Input: part model. Units: mm. Frame: model coordinates. A direction names the side the tool comes from. Coordinates: 2 decimals unless noted, no trailing zeros. Loops run counter-clockwise (first coordinate to the right, second up) from the corner with the lowest first, then second, coordinate; pieces in that order, holes last. Notation, with made-up numbers: (17.25, -34) -> (71.25, -34) arc R16 cw to (71.25, -8) -> close; hole circle Ø1 at (61.5, -10). An arc over 180 degrees is marked (long way). Answer as a JSON object with one key per item and string values.
from build123d import *

# Parameters (mm, degrees)
BOSS_EXTRUDE1_DEPTH  = 13
CUT_EXTRUDE1_DEPTH   = 66.5
BOSS_EXTRUDE4_DEPTH  = 6.1
CUT_EXTRUDE2_DEPTH   = 6.1
BOSS_EXTRUDE6_DEPTH  = 2.5
BOSS_EXTRUDE7_DEPTH  = 2.5
BOSS_EXTRUDE8_DEPTH  = 19.1
BOSS_EXTRUDE12_DEPTH = 9.5
BOSS_EXTRUDE13_DEPTH = 2.5
CUT_EXTRUDE4_DEPTH   = 5
CUT_EXTRUDE5_DEPTH   = 6.5
BOSS_EXTRUDE14_DEPTH = 10
CUT_EXTRUDE7_DEPTH   = 13
CUT_EXTRUDE8_DEPTH   = 5
CUT_EXTRUDE9_DEPTH   = 5
BOSS_EXTRUDE15_DEPTH = 2


with BuildPart() as part:
    # 3DSketch1 → Boss-Extrude1 (new body)
    with BuildSketch(Plane(origin=(0, 0, 0), x_dir=(0.970570246541768, 0, 0.2408181814727695), z_dir=(0, 1, 0))):
        Polygon((0, 0), (64.542921395, 16.014409068), (68.516421389, 0), (3.973499994, -16.014409068), align=None)
    extrude(amount=BOSS_EXTRUDE1_DEPTH)

    # 3DSketch2 → Cut-Extrude1 (cut)
    with BuildSketch(Plane(origin=(0, 13, 3.5), x_dir=(0, -0.8073911222578979, 0.59001658934231), z_dir=(1, 0, 0))):
        Polygon((0, 0), (10.496084589, 7.670215661), (11.971126063, 5.651737856), (1.475041473, -2.018477806), align=None)
        Polygon((14.626200715, 2.018477806), (4.130116125, -5.651737856), (5.605157599, -7.670215661), (16.101242188, 0), align=None)
    extrude(amount=CUT_EXTRUDE1_DEPTH, mode=Mode.SUBTRACT)


with BuildPart() as cut_extrude1_piece_1:
    # of the separate pieces the step leaves, piece 1, a body of its own (cut_extrude1_pieces)
    add(part.part.solids().sort_by_distance((0, 0, 10.5))[0])



with BuildPart() as cut_extrude1_piece_2:
    # of the separate pieces the step leaves, piece 2, a body of its own (cut_extrude1_pieces)
    add(part.part.solids().sort_by_distance((0, 0, 16.5))[0])


with BuildPart() as cut_extrude1_piece_3:
    # of the separate pieces the step leaves, piece 3, a body of its own (cut_extrude1_pieces)
    add(part.part.solids().sort_by_distance((0, 0, 0))[0])


with BuildPart() as cut_extrude1_piece_1_1:
    add(cut_extrude1_piece_1.part)

    add(cut_extrude1_piece_2.part)  # Boss-Extrude4 merges Cut-Extrude1 piece 2

    add(cut_extrude1_piece_3.part)  # Boss-Extrude4 merges Cut-Extrude1 piece 3
    # 3DSketch3 → Boss-Extrude4 (add)
    with BuildSketch(Plane(origin=(0, 13, 0), x_dir=(0.970570246541768, 0, 0.2408181814727695), z_dir=(0, 1, 0))):
        Polygon((0, 0), (64.542921395, 16.014409068), (68.516421389, 0), (3.973499994, -16.014409068), align=None)
    extrude(amount=BOSS_EXTRUDE4_DEPTH)

    # 3DSketch4 → Cut-Extrude2 (cut)
    with BuildSketch(Plane(origin=(2.463625992, 19.1, 3.5), x_dir=(0.9882657761690827, 0, 0.15274408549243565), z_dir=(0, 1, 0))):
        Polygon((0, 0), (60.744465433, 9.388524874), (62.195534245, 0), (1.451068812, -9.388524874), align=None)
    extrude(amount=-CUT_EXTRUDE2_DEPTH, mode=Mode.SUBTRACT)

    # 3DSketch5 → Boss-Extrude6 (add)
    with BuildSketch(Plane(origin=(0, 13, 3.5), x_dir=(0, -0.38512437764181645, 0.9228646779165425), z_dir=(-1, 0, 0))):
        Polygon((0, 0), (0.564008213, -1.351519893), (1.526819157, -3.658681588), (3.833980852, -2.695870643), (2.871169908, -0.388708949), (2.307161695, 0.962810944), align=None)
        Polygon((6.460052745, 2.695870643), (7.024060958, 1.344350751), (7.986871902, -0.962810944), (10.294033597, 0), (9.331222653, 2.307161695), (8.76721444, 3.658681588), align=None)
    extrude(amount=-BOSS_EXTRUDE6_DEPTH)

    # 3DSketch6 → Boss-Extrude7 (add)
    with BuildSketch(Plane(origin=(66.5, 0, 13), x_dir=(0, 0.8073911222578979, -0.5900165893423102), z_dir=(-1, 0, 0))):
        Polygon((0, 0), (1.475041473, 2.018477806), (11.971126063, -5.651737856), (10.496084589, -7.670215661), align=None)
        Polygon((14.626200715, -2.018477806), (4.130116125, 5.651737856), (5.605157599, 7.670215661), (16.101242188, 0), align=None)
    extrude(amount=BOSS_EXTRUDE7_DEPTH)

    # 3DSketch7 → Boss-Extrude8 (add)
    with BuildSketch(Plane(origin=(66.5, 0, 0), x_dir=(0.7713732785400773, 0, 0.6363829547955637), z_dir=(0, 1, 0))):
        Polygon((0, 0), (15.427465571, 12.727659096), (25.927784325, 0), (10.500318754, -12.727659096), align=None)
    extrude(amount=BOSS_EXTRUDE8_DEPTH)

    # 3DSketch8 → Boss-Extrude12 (add)
    with BuildSketch(Plane(origin=(76.128891267, 13, 6), x_dir=(-0.9382075830120803, 0, 0.3460730142305674), z_dir=(0, 1, 0))):
        Polygon((0, 0), (1.557328564, 4.221934124), (-1.734607538, 5.436217903), (-3.291936102, 1.214283779), align=None)
    extrude(amount=BOSS_EXTRUDE12_DEPTH)

    # 3DSketch9 → Boss-Extrude13 (add)
    with BuildSketch(Plane(origin=(75.345809824, 22.5, 11.764688466), x_dir=(0.5846855732237681, 0, -0.8112599956018993), z_dir=(0, 1, 0))):
        Polygon((0, 0), (5.702652298, 4.10997528), (8.664764649, 0), (2.962112351, -4.10997528), align=None)
    extrude(amount=BOSS_EXTRUDE13_DEPTH)

    # 3DSketch11 → Cut-Extrude4 (cut)
    with BuildSketch(Plane(origin=(0, 0, 0), x_dir=(0.9822888340033693, 0, 0.18737301457867736), z_dir=(0, -1, 0))):
        Polygon((0, 0), (3.091654741, 16.207765761), (88.059638882, 0), (84.967984141, -16.207765761), align=None)
    extrude(amount=-CUT_EXTRUDE4_DEPTH, mode=Mode.SUBTRACT)

    # 3DSketch12 → Cut-Extrude5 (cut)
    with BuildSketch(Plane(origin=(86.5, 5, 0), x_dir=(0, 0.6496523275821462, 0.7602314471705968), z_dir=(1, 0, 0))):
        Polygon((0, 0), (12.543818878, 10.719263405), (21.703916697, 0), (9.160097819, -10.719263405), align=None)
    extrude(amount=-CUT_EXTRUDE5_DEPTH, mode=Mode.SUBTRACT)

    # 3DSketch13 → Boss-Extrude14 (add)
    with BuildSketch(Plane(origin=(79.637641528, 22.5, 10.5), x_dir=(0, -0.6028330891856902, -0.7978673239222407), z_dir=(-1, 0, 0))):
        Polygon((0, 0), (2.049632503, 2.712748901), (5.640035461, 0), (3.590402958, -2.712748901), align=None)
    extrude(amount=BOSS_EXTRUDE14_DEPTH)

    # 3DSketch14 → Cut-Extrude7 (cut)
    with BuildSketch(Plane(origin=(80.41197271, 22.5, 4.735311534), x_dir=(0, 0.3350889131315588, 0.9421865103557314), z_dir=(-1, 0, 0))):
        Polygon((0, 0), (0.837722283, 2.355466276), (7.460706404, 0), (6.622984121, -2.355466276), align=None)
    extrude(amount=CUT_EXTRUDE7_DEPTH, mode=Mode.SUBTRACT)

    # 3DSketch15 → Cut-Extrude8 (cut)
    with BuildSketch(Plane(origin=(79.637641528, 22.5, 10.5), x_dir=(0, -0.6028330891856902, -0.7978673239222407), z_dir=(-1, 0, 0))):
        Polygon((0, 0), (2.049632503, 2.712748901), (5.640035461, 0), (3.590402958, -2.712748901), align=None)
    extrude(amount=CUT_EXTRUDE8_DEPTH, mode=Mode.SUBTRACT)

    # 3DSketch16 → Cut-Extrude9 (cut)
    with BuildSketch(Plane(origin=(80, 19.1, 0), x_dir=(0, -0.6496523275821462, 0.7602314471705968), z_dir=(-1, 0, 0))):
        Polygon((0, 0), (12.543818878, 10.719263405), (21.703916697, 0), (9.160097819, -10.719263405), align=None)
    extrude(amount=CUT_EXTRUDE9_DEPTH, mode=Mode.SUBTRACT)

    # 3DSketch17 → Boss-Extrude15 (add)
    with BuildSketch(Plane(origin=(68.168662732, 22.5, 12.3202178), x_dir=(0.6981467055639471, 0, -0.7159547314671559), z_dir=(0, -1, 0))):
        Polygon((0, 0), (5.828183385, -5.683218296), (11.370042327, 0), (5.541858942, 5.683218296), align=None)
    extrude(amount=-BOSS_EXTRUDE15_DEPTH)


solid = cut_extrude1_piece_1_1.part
1. Section query A-A (x = 31). Return loops of the section in (y, z), plus the area to 3 significant figures.
Reply:
{"outline": "(5, 0) -> (19.1, 0) -> (19.1, 3.5) -> (5, 3.5) -> close; (5, 6) -> (13, 6) -> (13, 10.5) -> (5, 10.5) -> close; (5, 13) -> (19.1, 13) -> (19.1, 16.5) -> (5, 16.5) -> close", "area": "135 mm2"}
2. Pin query (flat end, axial travel): P1, Ø2, axis at x = 44, z = 6, coming from the +Y side; P2, Ø1.3, axis at y = 11.5, z = 12.5, coming from the +X side; P3, Ø1.7, axis at y = 20.5, z = 8.5, coming from the -X side; P4, Ø6, axis at x = 42.5, z = 11, coming from the -Y side. Return the tip coordinate at first contact, or that it passes through.
Reply:
{"P1": "stops at y = 13", "P2": "stops at x = 75", "P3": "stops at x = 69.64", "P4": "stops at y = 5"}
3. Access query for faces 1 (the face through (74.638, 21, 8)), 2 (the face through (2.5, 11, 5)), 3 (the face through (72, 22.5, 11)), 4 (the face through (75, 12, 8)). Directions: +Z, -Z, +X, -X, +Y, -Y. A direction counts if a zero-diameter tool reaches every point of the face in a straight line with its end or side. Return the directions, or none.
Reply:
{"face 1": "+Z, -Z, +X", "face 2": "+Y, -Y", "face 3": "none", "face 4": "+Z, -Z, +X, -Y"}
4. Section query B-B (z = 8.75). Return loops of the section in (x, y), plus the area to 3 significant figures.
Reply:
{"outline": "(0, 5) -> (75, 5) -> (75, 19.1) -> (74.64, 19.1) -> (74.64, 22.5) -> (76.11, 22.5) -> (76.11, 24.5) -> (68.17, 24.5) -> (68.17, 22.5) -> (69.64, 22.5) -> (69.64, 19.1) -> (63.93, 19.1) -> (63.93, 13) -> (2.46, 13) -> (2.46, 19.1) -> (0, 19.1) -> close", "area": "715 mm2"}
5. Section query D-D (y = 14.25). Return loops of the section in (x, z).
Reply:
{"outline": "(0, 0) -> (75, 0) -> (75, 16.5) -> (0, 16.5) -> close; hole (2.46, 3.5) -> (63.93, 3.5) -> (63.93, 13) -> (2.46, 13) -> close"}
6. Section query C-C (x = 71.5). Return loops of the section in (y, z), plus the area to 3 significant figures.
Reply:
{"outline": "(5, 0) -> (19.1, 0) -> (19.1, 6) -> (22.5, 6) -> (22.5, 4.18) -> (24.5, 4.18) -> (24.5, 12.32) -> (22.5, 12.32) -> (22.5, 10.5) -> (19.1, 10.5) -> (19.1, 16.5) -> (5, 16.5) -> close", "area": "264 mm2"}
7. Mould query, pull axis X, two halves, no side actions, for faces 5 (the face through (2.5, 11, 12)), 6 (the face through (72, 23, 4.18)), 7 (the face through (69.638, 21, 8)). Classes: pulls with the +X half, pulls with the -X half, needs draft (parallel to the pull), parting line crosses it, or undercut.
Reply:
{"face 5": "undercut", "face 6": "needs draft", "face 7": "pulls with the -X half"}
8. Line query: line 1 along Z through (x, y) = (50.5, 11); line 2 along Z through (x, y) = (20, 18); line 3 along X through (y, z) = (17.5, 3.75). Output: solid intervals per line, ascending.
Reply:
{"line 1": "z = 0 to 3.5, 6 to 10.5, 13 to 16.5", "line 2": "z = 0 to 3.5, 13 to 16.5", "line 3": "x = 0 to 2.46, 63.93 to 75"}
